Input: dimensioned drawing with shaded views. Units: mm. Origin: part minimum x, y, z. A direction names the side the tool comes from. Coordinates: 2 decimals unless noted, no trailing zeros. Order: outer loops, then holes, each group sorted by start corner. A loop starts at its lowest first (then second) coordinate and runs counter-clockwise, first axis right, second up.
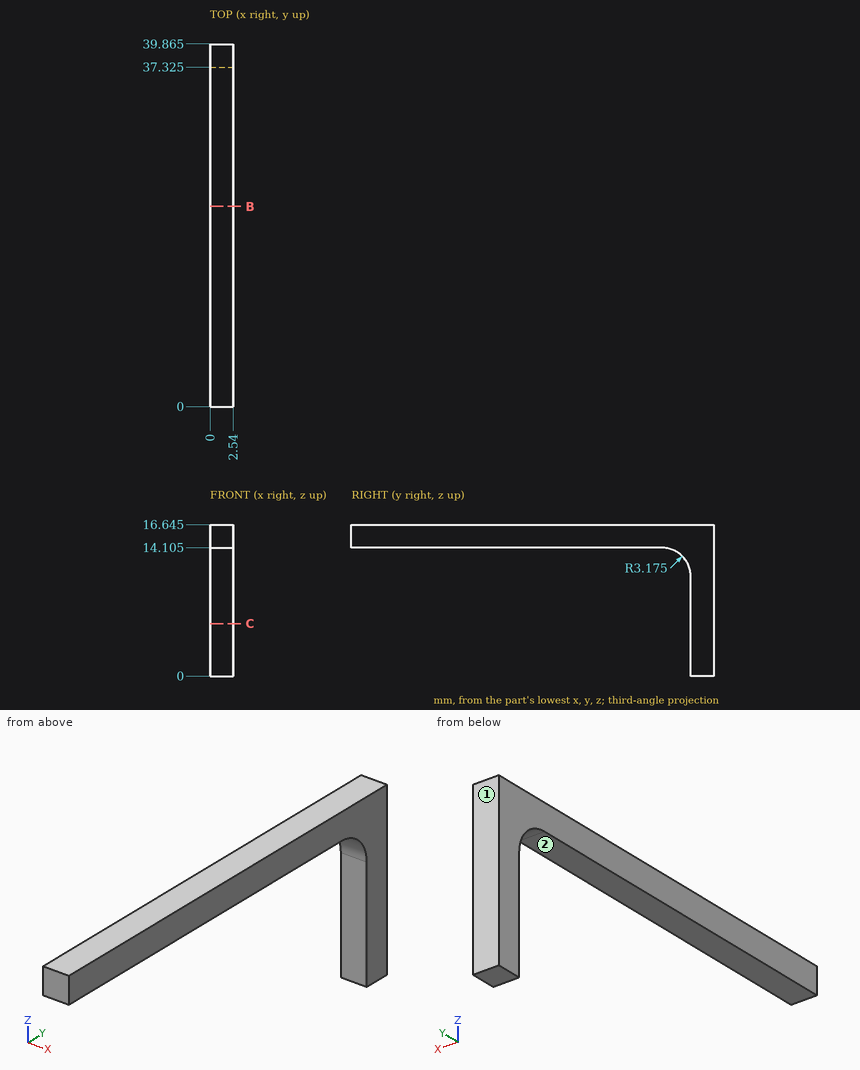
1. Access query for the marked faces 1 and 2. Directions: +Z, -Z, +X, -X, +Y, -Y. A direction counts if a zero-diameter tool reaches every point of the face in a straight line with its end or side. Return the directions, or none.
Findings:
face 1: +Z, -Z, +X, -X, +Y
face 2: -Z, +X, -X, -Y
2. Pin query (flat end, axial travel): P1, Ø0.8, axis at x = 2, y = 14, coming from the -Z side (1 decimal); P2, Ø5, axis at y = 12, z = 11, coming from the +X side. Return the tip coordinate at first contact, or that it passes through.
Findings:
P1: stops at z = 14.1
P2: passes through
3. Ray query, line 1 (Z direction, x = 0.65, y = 3.5) (1 decimal); line 2 (Y direction, x = 0.95, z = 1.5) (1 decimal); line 3 (Z direction, x = 0.2, y = 36) (1 decimal). Return the intervals inside material, ascending.
Findings:
line 1: z = 14.1 to 16.6
line 2: y = 37.3 to 39.9
line 3: z = 13.5 to 16.6
4. Section query C-C on z = 5.75. Return loops of the section in (x, y) (1 decimal).
Findings:
outline: (0, 37.3) - (2.5, 37.3) - (2.5, 39.9) - (0, 39.9) - close
5. Section query B-B on y = 22. Return loops of the section in (x, z) (1 decimal).
Findings:
outline: (0, 14.1) - (2.5, 14.1) - (2.5, 16.6) - (0, 16.6) - close
